Model file for the job. Use its own axes, mm. Face numbers are marked on the shaded views. A direction names the side the tool comes from. Give positions to 0.01 mm unless a question says otherwise; leave off trailing zeros. Order: outer loops, then holes, each group sorted by start corner. A loop starts at its lowest first (then second) coordinate and runs counter-clockwise, first axis right, second up. Notation, with made-up numbers: M 33.5,55 L 43.5,55 A34 cw 43.5,92 Z; hole C 4,76.25 d3. An arc over 180 degrees is marked long. Return JSON: item names as keys, results as strings. Group by question number.
1. Pin check, flat tips, straight feed: pin 1 (5 mm diameter, centred on x = 16, y = -6, fed in from +Z); pin 2 (2 mm diameter, centred on x = -9, z = 9.5, fed in from +Y); pin 3 (4 mm diameter, centred on y = -9, z = 6.5, fed in from -X); pin 4 (4 mm diameter, centred on x = -9, y = -1.5, fed in from -Z). Stop position of each tip, or through.
2. Wall check: probe 1 along Y at (x, z) = (0, 4.75); probe 2 along Z at (x, y) = (17, 8.5); probe 3 along X at (y, z) = (15, 7). Give the ranges that are in metal, low to high. Write a range as [from, to].
3. Slice it at C-C on y = -18. List the corners of the cut face in (x, z).
4. Slice it at A-A on z = 2.25. List the corners of the cut face in (x, y), then the cut area to 3 significant figures.
5. 3-axis set-ups, long thin cutter, end or side, ignore diameter. For the marked faces 5 and 6: which of +Z, -Z, +X, -X, +Y, -Y reach the whole face in a straight line?
6. Two-plate mould, pull along Y, no slides. Class the marked faces 1, 2, 3 and 4: released by +Y, released by -Y, zero draft, split by the parting line, or undercut.
7. Slice it at B-B on x = -1.5. List the corners of the cut face in (y, z).
8. Slice it at D-D on z = 16.75. List the corners of the cut face in (x, y).
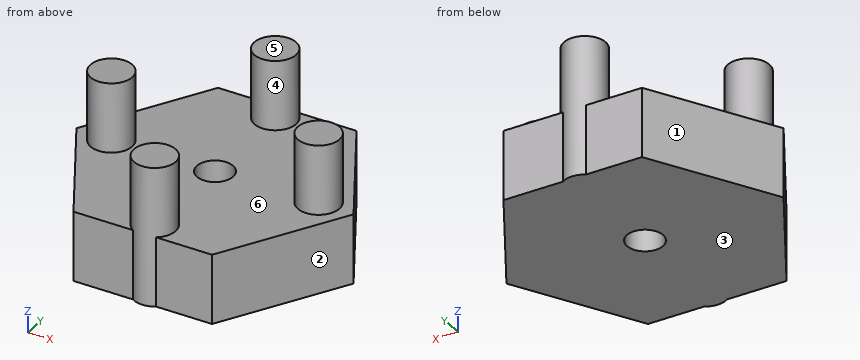
from build123d import *

# Parameters (mm, degrees)
F0_R     = 3.81
F1_DEPTH = 12.7
F2_R     = 3.302
F3_DEPTH = 25.4
F4_DEPTH = 25.4


# Not quite as in the source:
# - a feature names something its author has since deleted; it is built from what else it names


with BuildPart() as f1:
    # F0 (on Top) → F1 (new body)
    with BuildSketch(Plane.XY):
        with BuildLine():
            Line((2.1058679478, -22.0272163702), (12.4043320804, -22.1651200231))
            Line((12.4043320804, -22.1651200231), (25.3977230582, -0.3400933129))
            Line((25.3977230582, -0.3400933129), (12.9933909777, 21.8250267102))
            Line((12.9933909777, 21.8250267102), (2.1058679478, 21.9708182746))
            ThreePointArc((2.1058679478, 21.9708182746), (3.3265702822, 20.6034553453), (3.7674883359, 18.8243019401))
            ThreePointArc((3.7674883359, 18.8243019401), (-1.8666159044, 15.4793439852), (-2.1058679478, 22.0272163702))
            Line((-2.1058679478, 22.0272163702), (-12.4043320804, 22.1651200231))
            Line((-12.4043320804, 22.1651200231), (-25.3977230582, 0.3400933129))
            Line((-25.3977230582, 0.3400933129), (-12.9933909777, -21.8250267102))
            Line((-12.9933909777, -21.8250267102), (-2.1058679478, -21.9708182746))
            ThreePointArc((-2.1058679478, -21.9708182746), (-1.7366417411, -15.4552199938), (3.8525116641, -18.8243019401))
            ThreePointArc((3.8525116641, -18.8243019401), (3.3874696191, -20.6484061804), (2.1058679478, -22.0272163702))
        make_face()
        with Locations((-18.8243019401, -0.0425116641)):
            Circle(F0_R, mode=Mode.SUBTRACT)
        with Locations((18.8243019401, 0.0425116641)):
            Circle(F0_R, mode=Mode.SUBTRACT)
        with BuildLine():
            ThreePointArc((-2.1058679478, -21.9708182746), (-0.0085023328, -22.6339603988), (2.1058679478, -22.0272163702))
            Line((2.1058679478, -22.0272163702), (-2.1058679478, -21.9708182746))
        make_face()
        with BuildLine():
            Line((-2.1058679478, -21.9708182746), (2.1058679478, -22.0272163702))
            ThreePointArc((2.1058679478, -22.0272163702), (3.3874696191, -20.6484061804), (3.8525116641, -18.8243019401))
            ThreePointArc((3.8525116641, -18.8243019401), (-1.7366417411, -15.4552199938), (-2.1058679478, -21.9708182746))
        make_face()
        with BuildLine():
            ThreePointArc((3.7674883359, 18.8243019401), (3.3265702822, 20.6034553453), (2.1058679478, 21.9708182746))
            Line((2.1058679478, 21.9708182746), (-2.1058679478, 22.0272163702))
            ThreePointArc((-2.1058679478, 22.0272163702), (-1.8666159044, 15.4793439852), (3.7674883359, 18.8243019401))
        make_face()
        with BuildLine():
            Line((-2.1058679478, 22.0272163702), (2.1058679478, 21.9708182746))
            ThreePointArc((2.1058679478, 21.9708182746), (0.0085023328, 22.6339603988), (-2.1058679478, 22.0272163702))
        make_face()
    extrude(amount=F1_DEPTH)

    # F2 (on face) → F3 (cut)
    with BuildSketch(Plane.XY.offset(12.7)):
        Circle(F2_R)
    extrude(amount=-F3_DEPTH, mode=Mode.SUBTRACT)

    # F0 (on Top) → F4 (join)
    with BuildSketch(Plane.XY):
        with BuildLine():
            Line((-2.1058679478, 22.0272163702), (2.1058679478, 21.9708182746))
            ThreePointArc((2.1058679478, 21.9708182746), (0.0085023328, 22.6339603988), (-2.1058679478, 22.0272163702))
        make_face()
        with BuildLine():
            ThreePointArc((3.7674883359, 18.8243019401), (3.3265702822, 20.6034553453), (2.1058679478, 21.9708182746))
            Line((2.1058679478, 21.9708182746), (-2.1058679478, 22.0272163702))
            ThreePointArc((-2.1058679478, 22.0272163702), (-1.8666159044, 15.4793439852), (3.7674883359, 18.8243019401))
        make_face()
        with Locations((18.8243019401, 0.0425116641)):
            Circle(F0_R)
        with BuildLine():
            ThreePointArc((-2.1058679478, -21.9708182746), (-0.0085023328, -22.6339603988), (2.1058679478, -22.0272163702))
            Line((2.1058679478, -22.0272163702), (-2.1058679478, -21.9708182746))
        make_face()
        with BuildLine():
            Line((-2.1058679478, -21.9708182746), (2.1058679478, -22.0272163702))
            ThreePointArc((2.1058679478, -22.0272163702), (3.3874696191, -20.6484061804), (3.8525116641, -18.8243019401))
            ThreePointArc((3.8525116641, -18.8243019401), (-1.7366417411, -15.4552199938), (-2.1058679478, -21.9708182746))
        make_face()
        with Locations((-18.8243019401, -0.0425116641)):
            Circle(F0_R)
    extrude(amount=F4_DEPTH)


solid = f1.part
Result:
{
 "1": {"pin 1": "stops at z = 12.7", "pin 2": "stops at y = 22.13", "pin 3": "stops at x = -21.29", "pin 4": "stops at z = 0"},
 "2": {"probe 1": "y = [-22.63, -3.3], [3.3, 22.63]", "probe 2": "z = [0, 12.7]", "probe 3": "x = [-16.67, 16.81]"},
 "3": {"outline": "M -15.13,0 L 14.88,0 L 14.88,12.7 L 3.76,12.7 L 3.76,25.4 L -3.68,25.4 L -3.68,12.7 L -15.13,12.7 Z"},
 "4": {"outline": "M -25.4,0.34 L -12.99,-21.83 L -2.11,-21.97 A3.81 ccw 2.11,-22.03 L 12.4,-22.17 L 25.4,-0.34 L 12.99,21.83 L 2.11,21.97 A3.81 ccw -2.11,22.03 L -12.4,22.17 Z; hole C 0,0 d6.6", "area": "1,650 mm2"},
 "5": {"face 5": "+Z, +X, -X, +Y, -Y", "face 6": "+Z"},
 "6": {"face 1": "released by +Y", "face 2": "released by -Y", "face 3": "zero draft", "face 4": "undercut"},
 "7": {"outline": "M -22.31,0 L -2.94,0 L -2.94,12.7 L -15.34,12.7 L -15.34,25.4 L -22.31,25.4 Z; M 2.94,0 L 22.34,0 L 22.34,25.4 L 15.3,25.4 L 15.3,12.7 L 2.94,12.7 Z"},
 "8": {"outline": "C -18.82,-0.04 d7.62; C -0.04,18.82 d7.62; C 0.04,-18.82 d7.62; C 18.82,0.04 d7.62"}
}
